Read the model definition and answer for the solid it produces. Units are mm, in the model's axes. Round coordinates to 2 decimals unless told otherwise and drop trailing zeros. Order: outer loops, then holes, each group sorted by start corner. A loop starts at its lowest first (then second) coordinate and runs counter-clockwise, first axis right, second up. Notation, with made-up numbers: (-3.75, 22) - (6.25, 22) arc R24 ccw to (6.25, 36) - close; hole circle Ø9 at (49, 46). An arc over 180 degrees is marked (long way). Put each result on its own line as item: value. Start each with the question number.
Q1. For a pull along X with two mould halves and no side action, classify faces 1 (the face through (-47, 0, 1)), 2 (the face through (-1, 0, 3)), 3 (the face through (41.002, -1.245, 1.521)), 4 (the face through (47, 0, 1)) as pulls with the +X half, pulls with the -X half, needs draft (parallel to the pull), parting line crosses it, or undercut.
Q2. Section A-A on x = -38 is taken. Give the vertices of the cut face in (y, z), then the cut area to 3 significant figures.
Q3. Section C-C on z = 2.3 is taken. Give the vertices of the cut face in (x, y), then the cut area to 3 significant figures.
Q4. Find the intervals of material crossed by line 1 along Y through (x, z) = (-38, 1.9); line 2 along X through (y, z) = (-3, 1.85); line 3 along X through (y, z) = (-1.25, 2.55), in increasing order. Write a range as from..to.
Q5. Section B-B on y = 0 is taken. Give the vertices of the cut face in (x, z).
from build123d import *

# Parameters (mm, degrees)
CROQUIS1_W              = 94
CROQUIS1_H              = 15
SALIENTE_EXTRUIR1_DEPTH = 3
CORTAR_EXTRUIR1_REACH   = 49.689
CROQUIS2_R              = 3.25


with BuildPart() as part:
    # Croquis1 → Saliente-Extruir1 (new body)
    with BuildSketch(Plane.XY):
        Rectangle(CROQUIS1_W, CROQUIS1_H)
    extrude(amount=SALIENTE_EXTRUIR1_DEPTH)

    # Croquis2 → Cortar-Extruir1 (cut, up to next)
    with BuildSketch(Plane.XY.offset(3), mode=Mode.PRIVATE) as cortar_extruir1_sk1:
        with Locations((-38, 0)):
            Circle(CROQUIS2_R)
    cortar_extruir1_tool1 = extrude(cortar_extruir1_sk1.sketch, amount=-CORTAR_EXTRUIR1_REACH, mode=Mode.PRIVATE) & part.part
    # Croquis2 → Cortar-Extruir1 (cut, up to next)
    with BuildSketch(Plane.XY.offset(3), mode=Mode.PRIVATE) as cortar_extruir1_sk2:
        with Locations((38, 0)):
            Circle(CROQUIS2_R)
    cortar_extruir1_tool2 = extrude(cortar_extruir1_sk2.sketch, amount=-CORTAR_EXTRUIR1_REACH, mode=Mode.PRIVATE) & part.part
    add(cortar_extruir1_tool1.solids().sort_by_distance((-38, 0, 3))[0], mode=Mode.SUBTRACT)
    add(cortar_extruir1_tool2.solids().sort_by_distance((38, 0, 3))[0], mode=Mode.SUBTRACT)


solid = part.part
Findings:
1. face 1: pulls with the -X half
1. face 2: needs draft
1. face 3: undercut
1. face 4: pulls with the +X half
2. outline: (-7.5, 0) - (-3.25, 0) - (-3.25, 3) - (-7.5, 3) - close; (3.25, 0) - (7.5, 0) - (7.5, 3) - (3.25, 3) - close
2. area: 25.5 mm2
3. outline: (-47, -7.5) - (47, -7.5) - (47, 7.5) - (-47, 7.5) - close; hole circle Ø6.5 at (-38, 0); hole circle Ø6.5 at (38, 0)
3. area: 1,340 mm2
4. line 1: -7.5..-3.25, 3.25..7.5
4. line 2: -47..-39.25, -36.75..36.75, 39.25..47
4. line 3: -47..-41, -35..35, 41..47
5. outline: (-47, 0) - (-41.25, 0) - (-41.25, 3) - (-47, 3) - close; (-34.75, 0) - (34.75, 0) - (34.75, 3) - (-34.75, 3) - close; (41.25, 0) - (47, 0) - (47, 3) - (41.25, 3) - close
